from build123d import *

# Parameters (mm, degrees)
SKETCH1_R         = 48.5
SKETCH1_R_2       = 32.5
BODY_DEPTH        = 5
SKETCH2_R         = 5
BOLT_HOLE_DEPTH   = 69.771360318
CIRPATTERN1_COUNT = 12


with BuildPart() as part:
    # Sketch1 → Body (new body)
    with BuildSketch(Plane.XY):
        Circle(SKETCH1_R)
        Circle(SKETCH1_R_2, mode=Mode.SUBTRACT)
    extrude(amount=BODY_DEPTH)

    # Sketch2 → Bolt Hole (cut, through all)
    with BuildSketch(Plane.XY.offset(5)):
        with Locations((0, 40.5)):
            Circle(SKETCH2_R)
    bolt_hole = extrude(amount=-BOLT_HOLE_DEPTH, mode=Mode.SUBTRACT)

    # CirPattern1: Bolt Hole ×12 about axis
    cirpattern1_axis = Axis((0, 0, 0), (0, 0, 1))
    for i in range(1, CIRPATTERN1_COUNT):
        add(bolt_hole.rotate(cirpattern1_axis, i * 360 / CIRPATTERN1_COUNT), mode=Mode.SUBTRACT)


solid = part.part
Work out the finished part from the listing and answer in its coordinate system (mm). Give positions to 0.01 mm unless a question says otherwise; leave off trailing zeros. Loops run counter-clockwise (first coordinate to the right, second up) from the corner with the lowest first, then second, coordinate; pieces in that order, holes last. Notation, with made-up numbers: (24, -35.5) - (52, -35.5) arc R25 cw to (52, -9.5) - close; hole circle Ø10 at (60.5, 24.25). An arc over 180 degrees is marked (long way). Answer in a Markdown table with one row per item. Add a question column.
Q1. Consider line 1 along Y through (x, z) = (0, 3.9); line 2 along X through (y, z) = (-2, 4.3); line 3 along Y through (x, z) = (-1, 2.9). Determine where each line is inside the solid, lowest interval first.
Q2. Determine the mould class of faces 1 (the cylindrical face through (22.38, -43.028, 2.465)), 2 (the cylindrical face through (-32.767, -24.686, 2.535)), 3 (the cylindrical face through (-24.686, 32.767, 2.535)), 4 (the flat face through (-33, 0, 0)) for opening direction X: released by +X, released by -X, zero draft, split by the parting line, or undercut.
Q3. The part is cut by section A-A (y = 0). Determine the outline of the cut face in (x, z), and give its area (3 significant figures).
Q4. Each of these flat-tipped pins is pushed along its axis until it touches: P1, Ø1.5, axis at x = -28.5, z = 0.5, coming from the -Y side; P2, Ø1, axis at y = 38.5, z = 3, coming from the +X side; P3, Ø2, axis at x = 9, z = 1, coming from the -Y side. Where does it stop, or does it pass through?
Q5. The part is cut by section C-C (z = 1.4). State how many separate pieces and enclosed holes the cut face has, and give its area (3 significant figures).
Q6. The part is cut by section D-D (y = 13.5). Determine the outline of the cut face in (x, z).
Solution:
| question | item | result |
|---|---|---|
| 1 | line 1 | y = -48.5 to -45.5, -35.5 to -32.5, 32.5 to 35.5, 45.5 to 48.5 |
| 1 | line 2 | x = -48.46 to -45.08, -35.92 to -32.44, 32.44 to 35.92, 45.08 to 48.46 |
| 1 | line 3 | y = -48.49 to -45.4, -35.6 to -32.48, 32.48 to 35.6, 45.4 to 48.49 |
| 2 | face 1 | split by the parting line |
| 2 | face 2 | undercut |
| 2 | face 3 | undercut |
| 2 | face 4 | zero draft |
| 3 | outline | (-48.5, 0) - (-45.5, 0) - (-45.5, 5) - (-48.5, 5) - close; (-35.5, 0) - (-32.5, 0) - (-32.5, 5) - (-35.5, 5) - close; (32.5, 0) - (35.5, 0) - (35.5, 5) - (32.5, 5) - close; (45.5, 0) - (48.5, 0) - (48.5, 5) - (45.5, 5) - close |
| 3 | area | 60.0 mm² |
| 4 | P1 | stops at y = -39.78 |
| 4 | P2 | stops at x = 30.14 |
| 4 | P3 | stops at y = -47.84 |
| 5 | separate pieces | 1 |
| 5 | enclosed holes | 13 |
| 5 | area | 3,130 mm² |
| 6 | outline | (-46.58, 0) - (-29.56, 0) - (-29.56, 5) - (-46.58, 5) - close; (29.56, 0) - (46.58, 0) - (46.58, 5) - (29.56, 5) - close |
